```python
from build123d import *

# Parameters (mm, degrees)
RESSALTO_EXTRUS_O1_DEPTH = 6
ESBO_O2_W                = 87.948383594
ESBO_O2_H                = 90.794457537
CORTE_EXTRUS_O1_DEPTH    = 10
FILETE1_R                = 10
FILETE2_R                = 1
ESBO_O3_W                = 6
ESBO_O3_H                = 20
RESSALTO_EXTRUS_O2_DEPTH = 6
FILETE3_R                = 1
ESBO_O4_W                = 6
ESBO_O4_H                = 9.607959318
CORTE_EXTRUS_O2_DEPTH    = 6
CORTE_EXTRUS_O4_DEPTH    = 413.403928206
ESBO_O7_R                = 2.75
RESSALTO_EXTRUS_O3_DEPTH = 6
FILETE5_R                = 1
FILETE6_R                = 10
ESBO_O9_W                = 65.01383902
ESBO_O9_H                = 118.32551617
ESBO_O9_W_2              = 62.115199348
ESBO_O9_H_2              = 131.353950202
CORTE_EXTRUS_O5_DEPTH    = 417.006009572
ESBO_O10_W               = 6
ESBO_O10_H               = 17
CORTE_EXTRUS_O6_DEPTH    = 390.532068305
ESBO_O11_W               = 365
ESBO_O11_H               = 12
RESSALTO_EXTRUS_O4_DEPTH = 6
ESBO_O12_W               = 25.4
ESBO_O12_H               = 56.170187659
RESSALTO_EXTRUS_O5_DEPTH = 6
CHANFRO1_SIZE            = 3
FILETE7_R                = 2
ESBO_O13_R               = 3
CORTE_EXTRUS_O7_DEPTH    = 414.796075668
ESBO_O14_W               = 154.34893278
ESBO_O14_H               = 36.016450872
CORTE_EXTRUS_O8_DEPTH    = 414.796075668
FILETE8_R                = 13


with BuildPart() as part:
    # Esboço1 → Ressalto-extrusão1 (new body)
    with BuildSketch(Plane.XY):
        Polygon((0, 103.5), (0, 180), (365, 180), (365, 103.5), (371, 103.5), (371, 4.5), (365, 4.5), (365, 0), (0, 0), (0, 4.5), (-6, 4.5), (-6, 103.5), align=None)
    extrude(amount=RESSALTO_EXTRUS_O1_DEPTH)

    # Esboço2 → Corte-extrusão1 (cut)
    with BuildSketch(Plane.XY.offset(6)):
        with Locations((62.547917061, 118.567416428)):
            Rectangle(ESBO_O2_W, ESBO_O2_H)
        with Locations((302.452082939, 118.567416428)):
            Rectangle(ESBO_O2_W, ESBO_O2_H)
    extrude(amount=-CORTE_EXTRUS_O1_DEPTH, mode=Mode.SUBTRACT)

    # Filete1
    filete1_edges = [part.edges().sort_by_distance(p)[0] for p in [
        (18.573725264, 73.170187659, 3),
        (18.573725264, 163.964645196, 3),
        (106.522108858, 163.964645196, 3),
        (106.522108858, 73.170187659, 3),
        (346.426274736, 163.964645196, 3),
        (346.426274736, 73.170187659, 3),
        (258.477891142, 73.170187659, 3),
        (258.477891142, 163.964645196, 3),
    ]]
    fillet(filete1_edges, radius=FILETE1_R)

    # Filete2
    filete2_edges = [part.edges().sort_by_distance(p)[0] for p in [
        (-6, 103.5, 3),
        (-6, 4.5, 3),
        (371, 4.5, 3),
        (371, 103.5, 3),
    ]]
    fillet(filete2_edges, radius=FILETE2_R)

    # Esboço3 → Ressalto-extrusão2 (add)
    with BuildSketch(Plane.XY.offset(6)):
        with Locations((-3, 153.964645196)):
            Rectangle(ESBO_O3_W, ESBO_O3_H)
        with Locations((368, 153.964645196)):
            Rectangle(ESBO_O3_W, ESBO_O3_H)
    extrude(amount=-RESSALTO_EXTRUS_O2_DEPTH)

    # Filete3
    filete3_edges = [part.edges().sort_by_distance(p)[0] for p in [
        (-6, 143.964645196, 3),
        (-6, 163.964645196, 3),
        (371, 163.964645196, 3),
        (371, 143.964645196, 3),
    ]]
    fillet(filete3_edges, radius=FILETE3_R)

    # Esboço4 → Corte-extrusão2 (cut)
    with BuildSketch(Plane(origin=(371, 0, 0), x_dir=(0, 0, -1), z_dir=(1, 0, 0))):
        with Locations((-3, 98.696020341)):
            Rectangle(ESBO_O4_W, ESBO_O4_H)
    extrude(amount=-CORTE_EXTRUS_O2_DEPTH, mode=Mode.SUBTRACT)

    # Esboço6 → Corte-extrusão4 (cut, through all)
    with BuildSketch(Plane.XY.offset(6)):
        Polygon((106.522108858, 118.567416428), (258.477891142, 118.567416428), (346.426274736, 153.964645196), (346.426274736, 180), (18.573725264, 180), (18.573725264, 153.964645196), align=None)
    extrude(amount=-CORTE_EXTRUS_O4_DEPTH, mode=Mode.SUBTRACT)

    # Esboço7 → Ressalto-extrusão3 (add, through all)
    # profile 1 of 2: a face of its own
    with BuildSketch(Plane.XY.offset(6)):
        with BuildLine():
            ThreePointArc((-5, 163.964645196), (-15, 153.964645196), (-5, 143.964645196))
            ThreePointArc((-5, 143.964645196), (-3.426448861, 153.964645196), (-5, 163.964645196))
        make_face()
        with Locations((-9, 153.964645196)):
            Circle(ESBO_O7_R, mode=Mode.SUBTRACT)
    # profile 2 of 2: a face of its own
    with BuildSketch(Plane.XY.offset(6)):
        with BuildLine():
            ThreePointArc((365, 163.964645196), (363.426448861, 153.964645196), (365, 143.964645196))
            ThreePointArc((365, 143.964645196), (375, 153.964645196), (365, 163.964645196))
        make_face()
        with Locations((369, 153.964645196)):
            Circle(ESBO_O7_R, mode=Mode.SUBTRACT)
    extrude(amount=-RESSALTO_EXTRUS_O3_DEPTH)

    # Filete5
    filete5_edges = [part.edges().sort_by_distance(p)[0] for p in [
        (365, 180, 3),
        (0, 180, 3),
    ]]
    fillet(filete5_edges, radius=FILETE5_R)

    # Filete6
    filete6_edges = [part.edges().sort_by_distance(p)[0] for p in [
        (106.522108858, 118.567416428, 3),
        (258.477891142, 118.567416428, 3),
    ]]
    fillet(filete6_edges, radius=FILETE6_R)

    # Esboço9 → Corte-extrusão5 (cut, through all)
    with BuildSketch(Plane.XY.offset(6)):
        with Locations((-3.933194246, 132.332945744)):
            Rectangle(ESBO_O9_W, ESBO_O9_H)
        with Locations((367.48387441, 138.84716276)):
            Rectangle(ESBO_O9_W_2, ESBO_O9_H_2)
    extrude(amount=-CORTE_EXTRUS_O5_DEPTH, mode=Mode.SUBTRACT)

    # Esboço10 → Corte-extrusão6 (cut, through all)
    with BuildSketch(Plane.XY.offset(6)):
        with Locations((-3, 8.5)):
            Rectangle(ESBO_O10_W, ESBO_O10_H)
        with Locations((368, 8.5)):
            Rectangle(ESBO_O10_W, ESBO_O10_H)
    extrude(amount=-CORTE_EXTRUS_O6_DEPTH, mode=Mode.SUBTRACT)

    # Esboço11 → Ressalto-extrusão4 (add, through all)
    with BuildSketch(Plane.XY.offset(6)):
        with Locations((182.5, -6)):
            Rectangle(ESBO_O11_W, ESBO_O11_H)
    extrude(amount=-RESSALTO_EXTRUS_O4_DEPTH)

    # Esboço12 → Ressalto-extrusão5 (add, through all)
    with BuildSketch(Plane.XY.offset(6)):
        with Locations((383.7, 45.08509383)):
            Rectangle(ESBO_O12_W, ESBO_O12_H)
        with Locations((-18.7, 45.08509383)):
            Rectangle(ESBO_O12_W, ESBO_O12_H)
    extrude(amount=-RESSALTO_EXTRUS_O5_DEPTH)

    # Chanfro1
    chanfro1_edges = [part.edges().sort_by_distance(p)[0] for p in [
        (396.4, 73.170187659, 3),
        (396.4, 17, 3),
        (-31.4, 17, 3),
        (-31.4, 73.170187659, 3),
    ]]
    chamfer(chanfro1_edges, length=CHANFRO1_SIZE)

    # Filete7
    filete7_edges = [part.edges().sort_by_distance(p)[0] for p in [
        (0, -12, 3),
        (365, -12, 3),
    ]]
    fillet(filete7_edges, radius=FILETE7_R)

    # Esboço13 → Corte-extrusão7 (cut, through all)
    with BuildSketch(Plane.XY.offset(6)):
        with Locations((-20.3, 62)):
            Circle(ESBO_O13_R)
        with Locations((-20.3, 28)):
            Circle(ESBO_O13_R)
        with Locations(Location((385.3, 28, 0), (0, 0, 180))):
            Circle(ESBO_O13_R)
        with Locations(Location((385.3, 62, 0), (0, 0, 180))):
            Circle(ESBO_O13_R)
    extrude(amount=-CORTE_EXTRUS_O7_DEPTH, mode=Mode.SUBTRACT)

    # Esboço14 → Corte-extrusão8 (cut, through all)
    with BuildSketch(Plane.XY.offset(6)):
        with Locations((183.696575248, 113.87702748)):
            Rectangle(ESBO_O14_W, ESBO_O14_H)
    extrude(amount=-CORTE_EXTRUS_O8_DEPTH, mode=Mode.SUBTRACT)

    # Filete8
    filete8_edges = [part.edges().sort_by_distance(p)[0] for p in [
        (106.522108858, 95.868802044, 3),
        (258.477891142, 95.868802044, 3),
    ]]
    fillet(filete8_edges, radius=FILETE8_R)


solid = part.part
```
Design review of the part built by this model. Coordinates are the model's own, in mm. Give positions to 0.01 mm unless a question says otherwise; leave off trailing zeros. Write each loop counter-clockwise with the first axis right and the second up, starting at its lowest first coordinate (ties: lowest second). Pieces come first, ordered by that corner, then holes. Notation, with made-up numbers: (-29, 54.5) - (5, 54.5) arc R12 cw to (5, 67.5) - close; hole circle Ø5 at (53.25, 47.5). An arc over 180 degrees is marked (long way). Return JSON: item names as keys, results as strings. Group by question number.
(1) We need section B-B, the plane y = -2. Give the boundary of the cut face in (x, z).
(2) We need section C-C, the plane x = 303.5. Give the boundary of the cut face in (y, z).
(3) We need section A-A, the plane z = 4.5. Give the number of separate pieces and of enclosed holes in the cut face, then the cut area to 3 significant figures.
(4) Insertion check: pin 1 (3 mm diameter, centred on y = 4.5, z = 4, fed in from +X); pin 2 (1.8 mm diameter, centred on y = 7, z = 3, fed in from -X); pin 3 (2 mm diameter, centred on y = 18, z = 2.5, fed in from -X). Each pin has a flat end and moves straight along its axis. Give the tip position at first contact, or say it passes through.
(5) To check wall thickness, follow probe 1 along Y at (x, z) = (385.3, 2.4); probe 2 along Y at (x, z) = (76.5, 0.5); probe 3 along X at (y, z) = (8, 3.25). State the ranges of each line that lie inside material, in increasing order.
Reported:
{
 "1": {"outline": "(0, 0) - (365, 0) - (365, 6) - (0, 6) - close"},
 "2": {"outline": "(-12, 0) - (73.17, 0) - (73.17, 6) - (-12, 6) - close"},
 "3": {"separate pieces": "1", "enclosed holes": "4", "area": "37,900 mm2"},
 "4": {"pin 1": "stops at x = 365", "pin 2": "stops at x = 0", "pin 3": "stops at x = -30.4"},
 "5": {"probe 1": "y = 17 to 25, 31 to 59, 65 to 73.17", "probe 2": "y = -12 to 73.17", "probe 3": "x = 0 to 365"}
}
